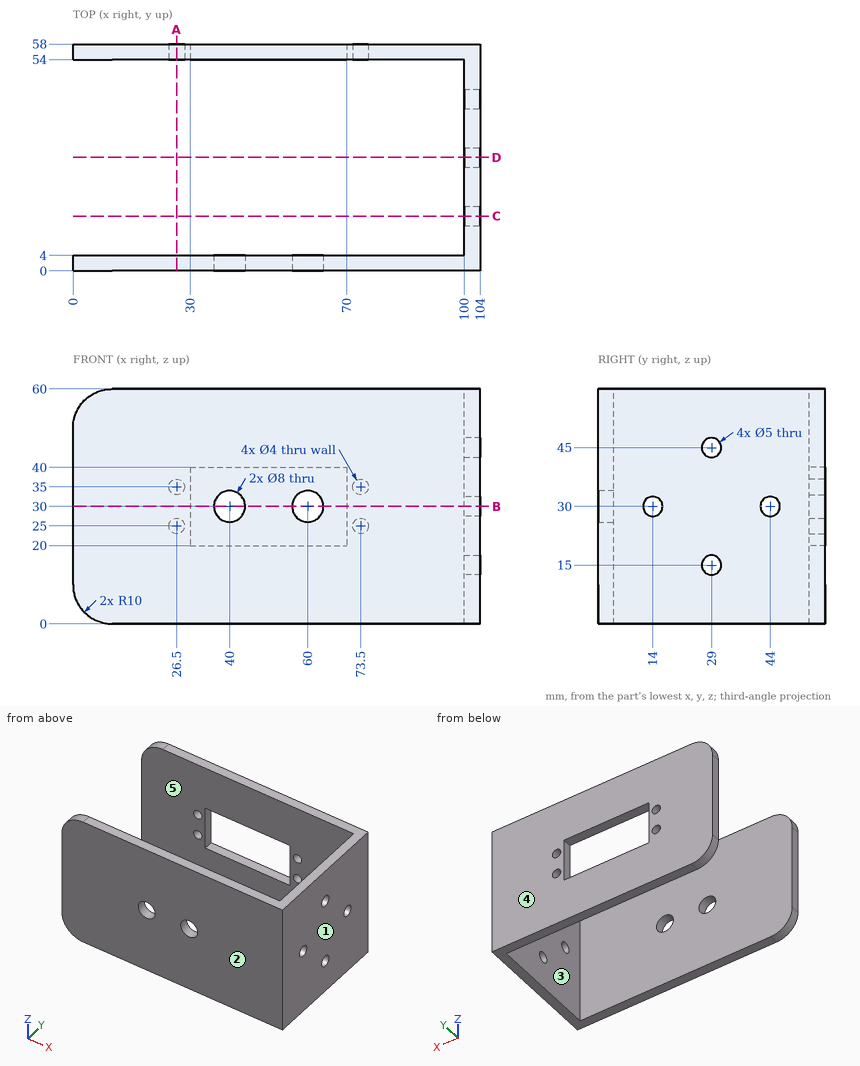
Answer from the drawing. Dimensions are ordinates in mm from the lowest x, y and z of the part. A direction names the side the tool comes from. Round coordinates to 2 decimals unless told otherwise and drop trailing zeros. Order: outer loops, then holes, each group sorted by start corner. A loop starts at its lowest first (then second) coordinate and runs counter-clockwise, first axis right, second up.
1) The part is cut by section B-B on z = 30. Write down the section's boundary in (x, y), plus the area to 3 significant figures.
2) For the marked faces 4 and 5, determine the directions among +Z, -Z, +X, -X, +Y, -Y from which every point of the face is accessible in a straight line to the end or side of a thin tool.
3) The mould has two halves that part along Y. Classify the marked faces 1, 2 and 3: released by +Y, released by -Y, zero draft, split by the parting line, or undercut.
4) Straight lines are drawn through the part: L1, parallel to X at y = 3, z = 30; L2, parallel to Z at x = 26.5, y = 56.3; L3, parallel to Y at x = 40.5, z = 16. For each, find the intervals that lie inside material, in ascending order.
5) The part is cut by section C-C on y = 14. Write down the section's boundary in (x, z), plus the area to 3 significant figures.
6) The part is cut by section A-A on x = 26.5. Write down the section's boundary in (y, z).
7) Flat-ended cylindrical pins translate along their axes: pin 1 (8 mm diameter, centred on y = 29, z = 15, fed in from -X); pin 2 (10.5 mm diameter, centred on x = 60, z = 30, fed in from +Y). Find the tip coordinate at first contact, or state that the pin passes through.
8) The part is cut by section D-D on y = 29. Write down the section's boundary in (x, z).
Resolved:
1. outline: (0, 0) - (36, 0) - (36, 4) - (0, 4) - close; (0, 54) - (30, 54) - (30, 58) - (0, 58) - close; (44, 0) - (56, 0) - (56, 4) - (44, 4) - close; (64, 0) - (104, 0) - (104, 11.5) - (100, 11.5) - (100, 4) - (64, 4) - close; (70, 54) - (100, 54) - (100, 46.5) - (104, 46.5) - (104, 58) - (70, 58) - close; (100, 16.5) - (104, 16.5) - (104, 41.5) - (100, 41.5) - close
1. area: 768 mm2
2. face 4: +Z, -Z, +X, -X, +Y
2. face 5: +Z, -Z, -X
3. face 1: zero draft
3. face 2: released by -Y
3. face 3: undercut
4. L1: x = 0 to 36, 44 to 56, 64 to 104
4. L2: z = 0 to 23, 27 to 33, 37 to 60
4. L3: y = 0 to 4, 54 to 58
5. outline: (100, 0) - (104, 0) - (104, 27.5) - (100, 27.5) - close; (100, 32.5) - (104, 32.5) - (104, 60) - (100, 60) - close
5. area: 220 mm2
6. outline: (0, 0) - (4, 0) - (4, 60) - (0, 60) - close; (54, 0) - (58, 0) - (58, 23) - (54, 23) - close; (54, 27) - (58, 27) - (58, 33) - (54, 33) - close; (54, 37) - (58, 37) - (58, 60) - (54, 60) - close
7. pin 1: stops at x = 100
7. pin 2: stops at y = 4
8. outline: (100, 0) - (104, 0) - (104, 12.5) - (100, 12.5) - close; (100, 17.5) - (104, 17.5) - (104, 42.5) - (100, 42.5) - close; (100, 47.5) - (104, 47.5) - (104, 60) - (100, 60) - close
